```python
from build123d import *

# Parameters (mm, degrees)
FILLET1_R = 2.54


with BuildPart() as part:
    # Sketch1 → Revolve1 (revolve)
    with BuildSketch(Plane(origin=(0, 0, 0), x_dir=(0, 0, -1), z_dir=(1, 0, 0))):
        with BuildLine():
            Line((0, 3.81), (0, 16.764))
            ThreePointArc((0, 16.764), (14.660113403, 14.487927839), (27.94, 7.874))
            Line((27.94, 7.874), (27.94, 1.524))
            Line((27.94, 1.524), (20.32, 1.524))
            Line((20.32, 1.524), (20.32, 0))
            Line((20.32, 0), (9.906, 0))
            Line((9.906, 0), (9.906, 3.81))
            Line((9.906, 3.81), (0, 3.81))
        make_face()
    revolve(axis=Axis((0, 3.81, 0), (0, 1, 0)))

    # Fillet1
    fillet1_edges = [part.edges().sort_by_distance(p)[0] for p in [
        (0, 7.874, 27.94),
        (0, 1.524, 27.94),
    ]]
    fillet(fillet1_edges, radius=FILLET1_R)


solid = part.part
```
Input: part model. Units: mm. Frame: model coordinates. Coordinates: 2 decimals unless noted, no trailing zeros. Write each loop counter-clockwise with the first axis right and the second up, starting at its lowest first coordinate (ties: lowest second). Pieces come first, ordered by that corner, then holes.
1) Material intervals for line 1 along Z through (x, y) = (0, 1.4); line 2 along X through (y, z) = (2.85, 0), sorted ascending.
2) Section A-A on y = 14.75. Output: boundary loops of the cut face in (x, z), and give its area (3 significant figures).
3) Section B-B on y = 2.75. Output: boundary loops of the cut face in (x, z).
4) Pin query (flat end, axial travel): pin 1 Ø10 at (x, y) = (15, 5) entering from -Z; pin 2 Ø12 at (x, z) = (9.5, 3.5) entering from +Y; pin 3 Ø10 at (x, z) = (-22, -13.5) entering from -Y. Return the tip coordinate at first contact, or that it passes through.
5) Section C-C on y = 9.5. Output: boundary loops of the cut face in (x, z), and give its area (3 significant figures).
6) Mould query, pull axis X, two halves, no side actions, for faces 1 (the cylindrical face through (-9.82, 1.93, 1.29)), 2 (the cylindrical face through (-27.7, 5.28, 3.64)), 3 (the flat face through (9, 0, 5)). Classes: pulls with the +X half, pulls with the -X half, needs draft (parallel to the pull), parting line crosses it, or undercut.
Check result:
1. line 1: z = -20.32 to -9.91, 9.91 to 20.32
1. line 2: x = -27.63 to -9.91, 9.91 to 27.63
2. outline: circle Ø27.62 at (0, 0)
2. area: 599 mm2
3. outline: circle Ø55.15 at (0, 0); hole circle Ø19.81 at (0, 0)
4. pin 1: stops at z = -26.09
4. pin 2: stops at y = 16.59
4. pin 3: stops at y = 1.52
5. outline: circle Ø50.98 at (0, 0)
5. area: 2,040 mm2
6. face 1: undercut
6. face 2: parting line crosses it
6. face 3: needs draft
